```python
from build123d import *

# Parameters (mm, degrees)
BOSS_EXTRUDE1_DEPTH = 10


# Read off the part's stored shape, not the designer's step: M3x0.5 Tapped Hole1
with BuildPart() as part:
    # Sketch1 → Boss-Extrude1 (new body)
    with BuildSketch(Plane(origin=(0, 0, 0), x_dir=(1, 0, 0), z_dir=(0, 1, 0))):
        with BuildLine():
            Line((-25, 4), (25, 4))
            ThreePointArc((25, 4), (29, 0), (25, -4))
            Line((25, -4), (-25, -4))
            ThreePointArc((-25, -4), (-29, 0), (-25, 4))
        make_face()
    extrude(amount=BOSS_EXTRUDE1_DEPTH)

    # M3x0.5 Tapped Hole1 outline → M3x0.5 Tapped Hole1 (revolve, cut)
    with BuildSketch(Plane(origin=(-25, 0, 0), x_dir=(1, 0, 0), z_dir=(0, 0, 1))):
        Polygon((0, 0), (1.25, 0), (1.25, 9.769247601), (1.525, 10), (0, 10), align=None)
    revolve(axis=Axis((-25, 0, 0), (0, 1, 0)), mode=Mode.SUBTRACT)

    # M3x0.5 Tapped Hole1 2 outline → M3x0.5 Tapped Hole1 2 (revolve, cut)
    with BuildSketch(Plane(origin=(25, 0, 0), x_dir=(1, 0, 0), z_dir=(0, 0, 1))):
        Polygon((0, 0), (1.25, 0), (1.25, 9.769247601), (1.525, 10), (0, 10), align=None)
    revolve(axis=Axis((25, 0, 0), (0, 1, 0)), mode=Mode.SUBTRACT)


solid = part.part
```
For this review, take the finished solid that the model builds, in its own axes (mm). Give positions to 0.01 mm unless a question says otherwise; leave off trailing zeros. Write each loop counter-clockwise with the first axis right and the second up, starting at its lowest first coordinate (ties: lowest second). Pieces come first, ordered by that corner, then holes.
Item 1: Take a section at A-A (z = 0). Give the boundary of the cut face in (x, y) (3 decimals), and give its area (3 significant figures).
Item 2: Take a section at C-C (z = 2.25). Give the boundary of the cut face in (x, y).
Item 3: Insertion check: P1, Ø4, axis at y = 5.5, z = -3, coming from the -X side. The pin has a flat end and moves straight along its axis. Give the tip position at first contact, or say it passes through.
Item 4: The part is to be moulded in two halves that separate along Z. For faces 1 (the face through (-23.845, 4.953, 0.479)), 2 (the face through (0, 5, 4)), 3 (the face through (0, 0, 0)), 4 (the face through (26.155, 4.953, 0.479)), say which applies: +Z half, -Z half, draft (parallel to the pull), parting line (faces both ways), or undercut.
Item 5: Take a section at B-B (y = 6). Give the boundary of the cut face in (x, z), and give its area (3 significant figures).
Item 6: Take a section at D-D (z = -2.75). Give the boundary of the cut face in (x, y).
Item 7: Wall thickness on probe 1 along X at (y, z) = (5.25, 0); probe 2 along Z at (x, y) = (25, 2.5); probe 3 along X at (y, z) = (7.5, -0.5): over which ranges is each line inside the solid? List them lowest first.
Established:
1. outline: (-29, 0) - (-26.25, 0) - (-26.25, 9.769) - (-26.525, 10) - (-29, 10) - close; (-23.75, 0) - (23.75, 0) - (23.75, 9.769) - (23.475, 10) - (-23.475, 10) - (-23.75, 9.769) - close; (26.25, 0) - (29, 0) - (29, 10) - (26.525, 10) - (26.25, 9.769) - close
1. area: 530 mm2
2. outline: (-28.31, 0) - (28.31, 0) - (28.31, 10) - (-28.31, 10) - close
3. P1: stops at x = -28.87
4. face 1: undercut
4. face 2: +Z half
4. face 3: draft
4. face 4: undercut
5. outline: (-25, -4) - (25, -4) arc R4 ccw to (25, 4) - (-25, 4) arc R4 ccw to start; hole circle Ø2.5 at (-25, 0); hole circle Ø2.5 at (25, 0)
5. area: 440 mm2
6. outline: (-27.9, 0) - (27.9, 0) - (27.9, 10) - (-27.9, 10) - close
7. probe 1: x = -29 to -26.25, -23.75 to 23.75, 26.25 to 29
7. probe 2: z = -4 to -1.25, 1.25 to 4
7. probe 3: x = -28.97 to -26.15, -23.85 to 23.85, 26.15 to 28.97
